Answer from the drawing. Dimensions are ordinates in mm from the lowest x, y and z of the part. Coordinates: 2 decimals unless noted, no trailing zeros. Order: outer loops, then holes, each group sorted by start corner. A loop starts at its lowest first (then second) coordinate and runs counter-clockwise, first axis right, second up. Notation, with made-up numbers: M 80.25,39.5 L 136.25,39.5 A24 cw 136.25,66.5 Z; hole C 64,4 d1. An arc over 180 degrees is marked long. One line per question, with ' | ' between items. Start each with the question number.
1) Find section A-A, the plane y = 33. Write down the section's boundary in (x, z), plus the area to 3 significant figures.
2) Find section B-B, the plane z = 20. Write down the section's boundary in (x, y), plus the area to 3 significant figures.
3) Find section C-C, the plane x = 1.55. Count the separate pieces of the cut face and the enclosed holes in it, plus the area to 3 significant figures.
4) Find section D-D, the plane z = 48.5. Write down the section's boundary in (x, y).
5) Consider probe 1 along Y at (x, z) = (0.7, 63); probe 2 along Y at (x, z) = (1.8, 20); probe 3 along Y at (x, z) = (0.65, 40.5). Determine where each line is inside the solid, lowest interval first.
6) Given P1, Ø1.5, axis at x = 1.5, z = 3, coming from the -Y side; P2, Ø0.9, axis at x = 2, y = 35, coming from the -Z side; P3, Ø0.9, axis at x = 2, y = 2, coming from the +Z side, each flat-ended and moving along its own axis, determine where each tip first touches the part or whether it passes through.
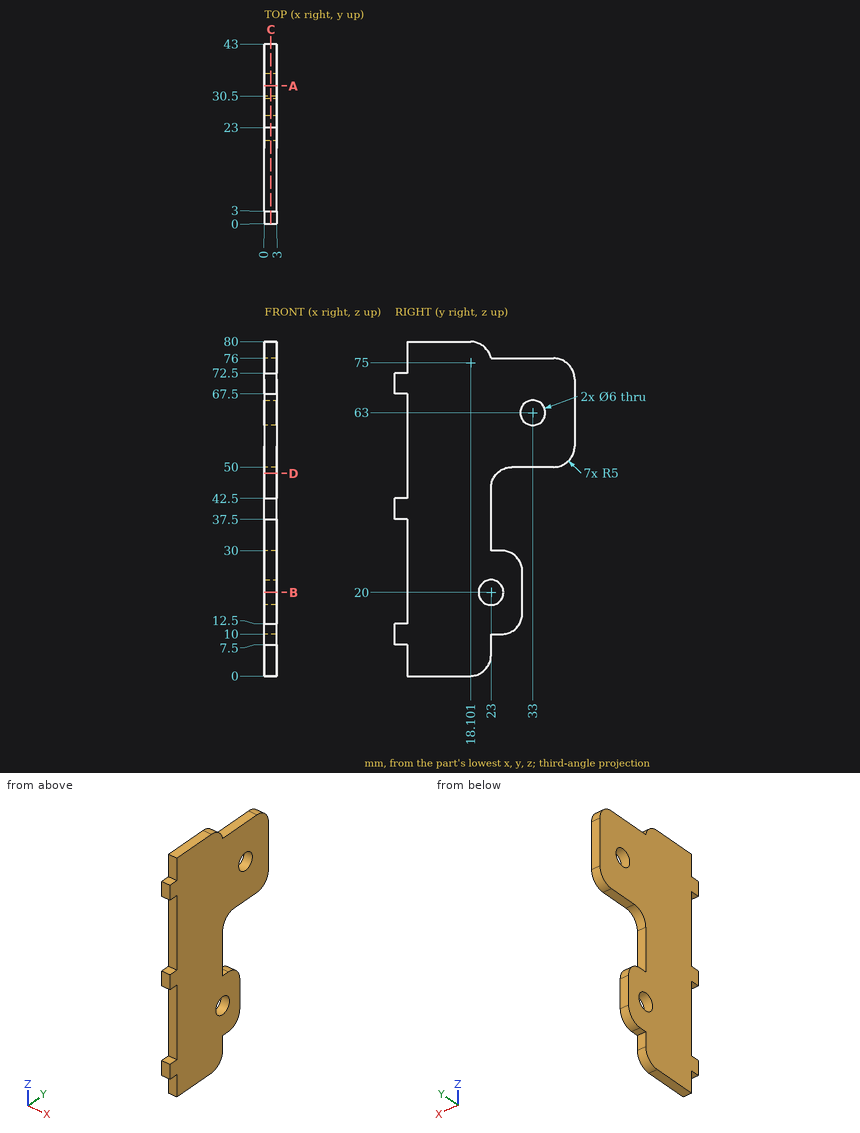
Report:
1) outline: M 0,50 L 3,50 L 3,60 L 0,60 Z; M 0,66 L 3,66 L 3,76 L 0,76 Z | area: 60.0 mm^2
2) outline: M 0,3 L 3,3 L 3,20 L 0,20 Z; M 0,26 L 3,26 L 3,30.5 L 0,30.5 Z | area: 64.5 mm^2
3) separate pieces: 1 | enclosed holes: 2 | area: 2,230 mm^2
4) outline: M 0,3 L 3,3 L 3,24.43 L 0,24.43 Z
5) probe 1: y = 3 to 30, 36 to 43 | probe 2: y = 3 to 20, 26 to 30.5 | probe 3: y = 0 to 23
6) P1: stops at y = 3 | P2: stops at z = 50 | P3: stops at z = 72.5
